The figure shows three views and two pictorial views of one solid part (mm, origin at its lowest corner). Answer the questions. A direction names the side the tool comes from. Round coordinates to 2 decimals unless told otherwise and drop trailing zeros. Write each loop counter-clockwise with the first axis right and the second up, starting at its lowest first coordinate (ties: lowest second). Pieces come first, ordered by that corner, then holes.
Item 1: Find section A-A on y = 3.83. Give the vertices of the cut face in (x, z).
Item 2: Find section B-B on z = 2.25. Give the vertices of the cut face in (x, y), then the cut area to 3 significant figures.
Item 3: A tool of negligible diameter and unlimited length cuts with its end or side. For the marked faces 1 and 2, from which of +Z, -Z, +X, -X, +Y, -Y can it reach the whole face along a straight path? Write none if from no direction.
Item 4: Find the intervals of material crossed by probe 1 along Z at (x, y) = (4, 1); probe 2 along Y at (x, z) = (2.75, 1.75); probe 3 along X at (y, z) = (2.5, 11.5) (1 decimal), in increasing order.
Item 5: Each of these flat-tipped pins is pushed along its axis until it touches: pin 1 (1.5 mm diameter, centred on x = 4.5, z = 4, fed in from -Y); pin 2 (1.5 mm diameter, centred on x = 2.5, z = 9, fed in from -Y); pin 3 (1 mm diameter, centred on y = 4, z = 9.5, fed in from +X). Where does it stop, or does it pass through?
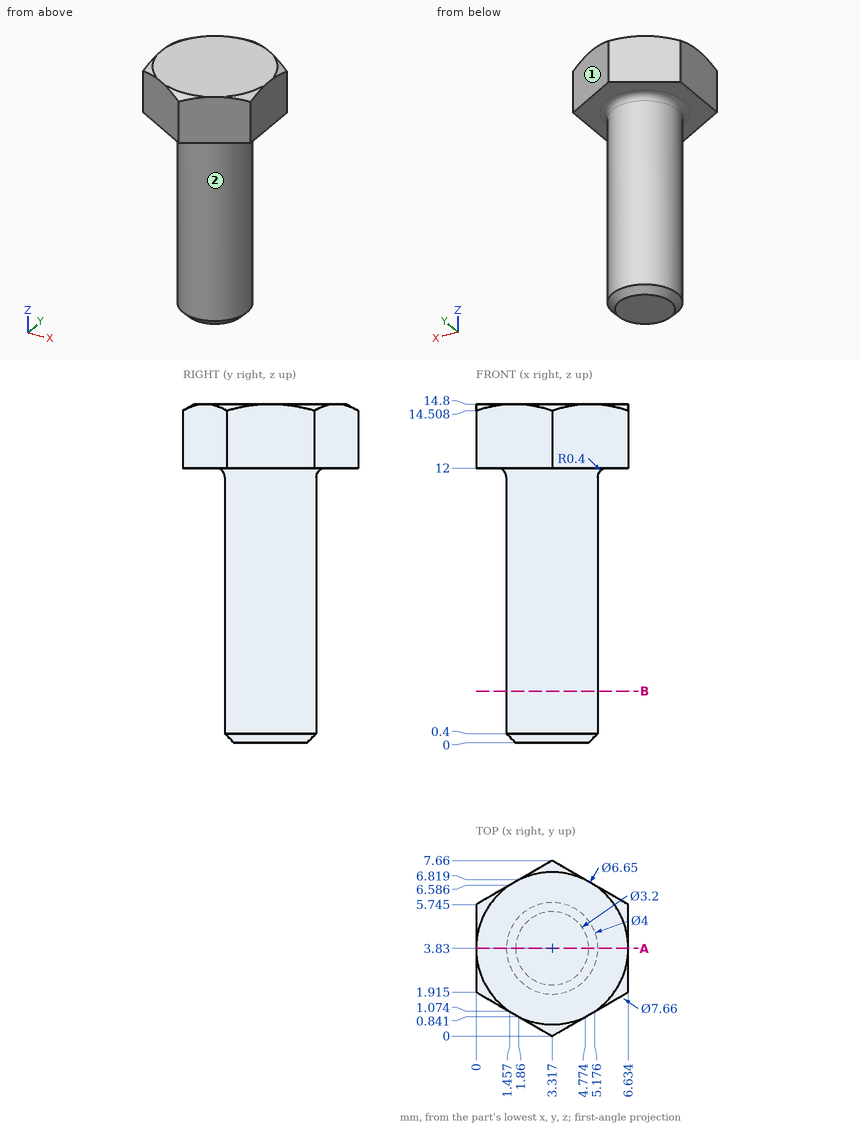
Check values:
1. outline: (0, 12) - (0.92, 12) arc R0.4 cw to (1.32, 11.6) - (1.32, 0.4) - (1.72, 0) - (4.92, 0) - (5.32, 0.4) - (5.32, 11.6) arc R0.4 cw to (5.72, 12) - (6.63, 12) - (6.63, 14.8) - (0, 14.8) - close
2. outline: circle Ø4 at (3.32, 3.83)
2. area: 12.6 mm2
3. face 1: +Z, -Z, +X, +Y
3. face 2: -Z
4. probe 1: z = 12 to 14.8
4. probe 2: y = 1.91 to 5.75
4. probe 3: x = 1.8 to 4.8
5. pin 1: stops at y = 1.88
5. pin 2: stops at y = 1.83
5. pin 3: stops at x = 5.32
